The drawing under review shows one solid part. Ordinate dimensions are in mm from its lowest x, y, z. A direction names the side the tool comes from. Coordinates: 2 decimals unless noted, no trailing zeros. Write each loop counter-clockwise with the first axis right and the second up, starting at its lowest first coordinate (ties: lowest second). Pieces come first, ordered by that corner, then holes. Notation, with made-up numbers: (63.25, 74) -> (71.25, 74) arc R12 cw to (71.25, 90) -> close; hole circle Ø11 at (40.25, 45.5). An arc over 180 degrees is marked (long way). One line per item, written item: value. Start each with the question number.
1) For probe 1 along X at (y, z) = (10.5, 6.25); probe 2 along Y at (x, z) = (10, 6.25); probe 3 along X at (y, z) = (14.5, 19.75), list the stretches that pass through material, from the lowest coordinate up. Write a range as from..to.
2) For pin 1 Ø10 at (y, z) = (5, 8.5) entering from +X; pin 2 Ø2 at (x, z) = (15.5, 3.5) entering from +Y; pin 3 Ø5 at (x, z) = (12.5, 8) entering from +Y (3 decimals), all flat-tipped, find the tip position at first contact; note any pin that passes through.
3) Add section B-B (x = 7.75). State the section outline as (y, z) points.
4) Add section D-D (x = 2.75). State the section outline as (y, z) points, and give its area (3 significant figures).
5) Add section A-A (y = 14.75). State the section outline as (x, z) points, and give its area (3 significant figures).
6) Machinability: for the marked faces 4 and 5, which of the approach directions +Z, -Z, +X, -X, +Y, -Y give a long, thin tool a straight path to every point of the face, cutting with its end or side? Answer none if there is none.
7) Mouldability with a two-part tool opening along X and no side actions: class the marked faces 1, 2 and 3 as released by +X, released by -X, zero draft, split by the parting line, or undercut.
8) Add section C-C (z = 4.5). State the section outline as (x, y) points (3 decimals).
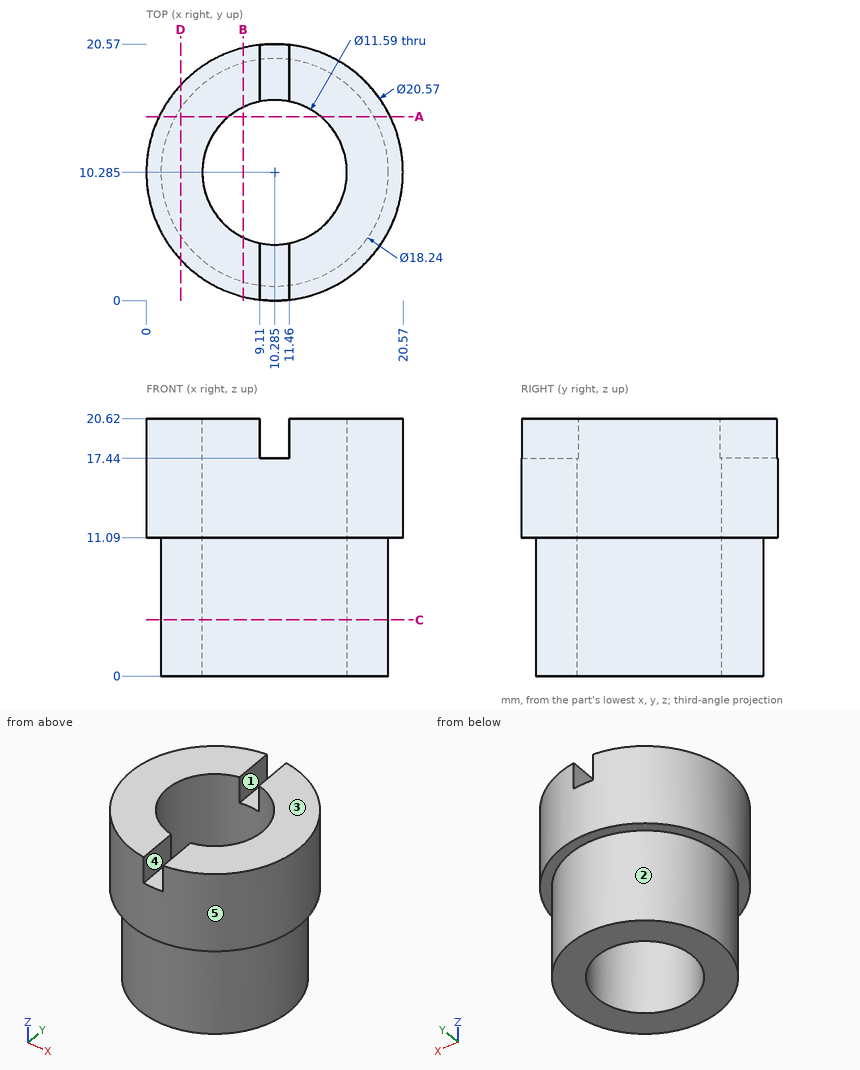
Numbers:
1. probe 1: 1.17..4.49, 16.08..19.4
1. probe 2: 1.17..4.5, 16.07..19.4
1. probe 3: 0.9..6.31, 14.26..19.67
2. pin 1: x = 20.52
2. pin 2: y = 18.37
2. pin 3: y = 19.405
3. outline: (0.32, 11.09) -> (1.52, 11.09) -> (1.52, 0) -> (5.07, 0) -> (5.07, 20.62) -> (0.32, 20.62) -> close; (15.5, 0) -> (19.05, 0) -> (19.05, 11.09) -> (20.25, 11.09) -> (20.25, 20.62) -> (15.5, 20.62) -> close
4. outline: (3.28, 11.09) -> (5.15, 11.09) -> (5.15, 0) -> (15.42, 0) -> (15.42, 11.09) -> (17.29, 11.09) -> (17.29, 20.62) -> (3.28, 20.62) -> close
4. area: 247 mm²
5. outline: (1.02, 11.09) -> (2.33, 11.09) -> (2.33, 0) -> (6.59, 0) -> (6.59, 20.62) -> (1.02, 20.62) -> close; (13.98, 0) -> (18.24, 0) -> (18.24, 11.09) -> (19.55, 11.09) -> (19.55, 20.62) -> (13.98, 20.62) -> close
5. area: 201 mm²
6. face 4: +Z, +Y, -Y
6. face 5: +Z, -Z
7. face 1: undercut
7. face 2: split by the parting line
7. face 3: zero draft
8. outline: circle Ø18.24 at (10.285, 10.285); hole circle Ø11.59 at (10.285, 10.285)
